from build123d import *

# Parameters (mm, degrees)
SKETCH2_W            = 123.19
SKETCH2_H            = 53.34
BOSS_EXTRUDE2_DEPTH  = 6.35
BOSS_EXTRUDE3_DEPTH  = 45.72
BOSS_EXTRUDE1_DEPTH  = 10
LPATTERN1_COUNT      = 5
LPATTERN1_PITCH      = 22.86
LPATTERN1_COUNT_DIR2 = 2
LPATTERN1_PITCH_DIR2 = 22.86
SKETCH6_R            = 2.75
CUT_EXTRUDE1_DEPTH   = 5.5


with BuildPart() as part:
    # Sketch2 → Boss-Extrude2 (new body)
    with BuildSketch(Plane(origin=(0, 0, 0), x_dir=(1, 0, 0), z_dir=(0, 1, 0))):
        Polygon((123.19, 53.34), (123.19, 0), (133.35, 0), (133.35, 63.5), (0, 63.5), (0, 53.34), align=None)
        with Locations((61.595, 26.67)):
            Rectangle(SKETCH2_W, SKETCH2_H)
    extrude(amount=BOSS_EXTRUDE2_DEPTH)

    # Sketch2_4 → Boss-Extrude3 (add)
    with BuildSketch(Plane(origin=(0, 0, 0), x_dir=(1, 0, 0), z_dir=(0, 1, 0))):
        Polygon((123.19, 53.34), (123.19, 0), (133.35, 0), (133.35, 63.5), (0, 63.5), (0, 53.34), align=None)
    extrude(amount=BOSS_EXTRUDE3_DEPTH)

    # Sketch1 → Boss-Extrude1 (add)
    with BuildSketch(Plane(origin=(0, 6.35, 6.35), x_dir=(1, 0, 0), z_dir=(0, 1, 0))):
        with BuildLine():
            Line((13.335, 31.115), (17.145, 31.115))
            ThreePointArc((17.145, 31.115), (22.533153673, 28.883153673), (24.765, 23.495))
            Line((24.765, 23.495), (24.765, 19.685))
            ThreePointArc((24.765, 19.685), (22.533153673, 14.296846327), (17.145, 12.065))
            Line((17.145, 12.065), (13.335, 12.065))
            ThreePointArc((13.335, 12.065), (7.946846327, 14.296846327), (5.715, 19.685))
            Line((5.715, 19.685), (5.715, 23.495))
            ThreePointArc((5.715, 23.495), (7.946846327, 28.883153673), (13.335, 31.115))
        make_face()
    boss_extrude1 = extrude(amount=BOSS_EXTRUDE1_DEPTH)

    # LPattern1: Boss-Extrude1 5 × 2
    with Locations(*[(i * LPATTERN1_PITCH, 0, -j * LPATTERN1_PITCH_DIR2) for i in range(LPATTERN1_COUNT) for j in range(LPATTERN1_COUNT_DIR2) if (i, j) != (0, 0)]):
        add(boss_extrude1)

    # Sketch6 → Cut-Extrude1 (cut)
    with BuildSketch(Plane(origin=(0, 16.35, 0), x_dir=(1, 0, 0), z_dir=(0, 1, 0))):
        with Locations(Location((106.354086264, 38.229532142, 0), (0, 0, 270))):
            Circle(SKETCH6_R)
        with Locations(Location((14.914086264, 38.229532142, 0), (0, 0, 270))):
            Circle(SKETCH6_R)
    extrude(amount=-CUT_EXTRUDE1_DEPTH, mode=Mode.SUBTRACT)


solid = part.part
Part model, mm, in its own coordinate system. A direction names the side the tool comes from. Coordinates: 2 decimals unless noted, no trailing zeros. Loops run counter-clockwise (first coordinate to the right, second up) from the corner with the lowest first, then second, coordinate; pieces in that order, holes last. Notation, with made-up numbers: (-18, -0.75) - (38, -0.75) arc R7 cw to (38, 7.25) - close; hole circle Ø10 at (-21, -10). An arc over 180 degrees is marked (long way). Write each question's results on one line, items separated by ' | '. Start each with the question number.
Q1. Drop flat-ended pins along their axis: pin 1 Ø5 at (x, z) = (78, -15) entering from +Y; pin 2 Ø1.1 at (y, z) = (13, -15) entering from -X (3 decimals); pin 3 Ø1.5 at (y, z) = (17.5, -18.5) entering from -X. Give the stop position or say it passes through.
Q2. Slice it at D-D on x = 10. Give the cut face in (y, z), and give its area (3 significant figures).
Q3. Which spindle directions (+Z, -Z, +X, -X, +Y, -Y) get a long thin tool onto all of the face, cutting with end or side? Do faces 1 (the cylindrical face through (30.866, 11.28, -7.888)), 2 (the flat face through (68, 23, -63.5)), 3 (the cylindrical face through (45.334, 11.28, -22.592)), 4 (the flat face through (84, 16.35, -38)), 5 (the flat face through (38, 11, -47.625)). Say none if no direction does.
Q4. Two-plate mould, pull along X, no slides. Class faces 6 (the flat face through (15, 11, -47.625)), 7 (the cylindrical face through (8.006, 11.28, -30.748)), 8 (the cylindrical face through (99.328, 11.28, -45.334)): +X half, -X half, draft (parallel to the pull), parting line (faces both ways), or undercut.
Q5. Slice it at B-B on x = 23.5. Give the cut face in (y, z).
Q6. Slice it at A-A on y = 24.5. Give the cut face in (x, z).
Q7. Probe line 1 along X through (y, z) = (15, -35); line 2 along X through (y, z) = (16, -10.5); line 3 along X through (y, z) = (28.5, -39). List the from-to ranges inside material, lowest first.
Answer:
1) pin 1: stops at y = 16.35 | pin 2: stops at x = 5.715 | pin 3: stops at x = 123.19
2) outline: (0, -63.5) - (45.72, -63.5) - (45.72, -53.34) - (6.35, -53.34) - (6.35, -46.86) - (16.35, -46.86) - (16.35, -29.34) - (6.35, -29.34) - (6.35, -24) - (16.35, -24) - (16.35, -6.48) - (6.35, -6.48) - (6.35, 0) - (0, 0) - close | area: 1,150 mm2
3) face 1: +Z, +Y | face 2: -Z, +X, -X, +Y, -Y | face 3: +Y | face 4: +Z, -X, +Y | face 5: -X, +Y
4) face 6: draft | face 7: -X half | face 8: undercut
5) outline: (0, -63.5) - (45.72, -63.5) - (45.72, -53.34) - (6.35, -53.34) - (6.35, -44.21) - (16.35, -44.21) - (16.35, -31.99) - (6.35, -31.99) - (6.35, -21.35) - (16.35, -21.35) - (16.35, -9.13) - (6.35, -9.13) - (6.35, 0) - (0, 0) - close
6) outline: (0, -63.5) - (133.35, -63.5) - (133.35, 0) - (123.19, 0) - (123.19, -53.34) - (0, -53.34) - close
7) line 1: x = 5.81 to 24.67, 28.67 to 47.53, 51.53 to 70.39, 74.39 to 93.25, 97.25 to 116.11, 123.19 to 133.35 | line 2: x = 6.26 to 24.22, 29.12 to 47.08, 51.98 to 69.94, 74.84 to 92.8, 97.7 to 115.66, 123.19 to 133.35 | line 3: x = 123.19 to 133.35
